Answer from the drawing. Dimensions are ordinates in mm from the lowest x, y and z of the part. Coordinates: 2 decimals unless noted, no trailing zeros. Write each loop counter-clockwise with the first axis right and the second up, starting at its lowest first coordinate (ties: lowest second). Pieces come first, ordered by that corner, then holes.
1) Determine the mould class of the marked faces 1, 2 and 3 for opening direction X: +X half, -X half, draft (parallel to the pull), parting line (faces both ways), or undercut.
2) The part is cut by section A-A (z = 1.75). Determine the outline of the cut face in (x, y).
3) Find the intervals of material crossed by line 1 (X direction, y = 0.25, z = 3.5) (1 decimal); line 2 (X direction, y = 1, z = 4); line 3 (Z direction, x = 3, y = 1.3) (1 decimal), in increasing order.
4) The part is cut by section D-D (z = 5.5). Determine the outline of the cut face in (x, y).
5) The part is cut by section B-B (x = 3.5). Determine the outline of the cut face in (y, z) (1 decimal).
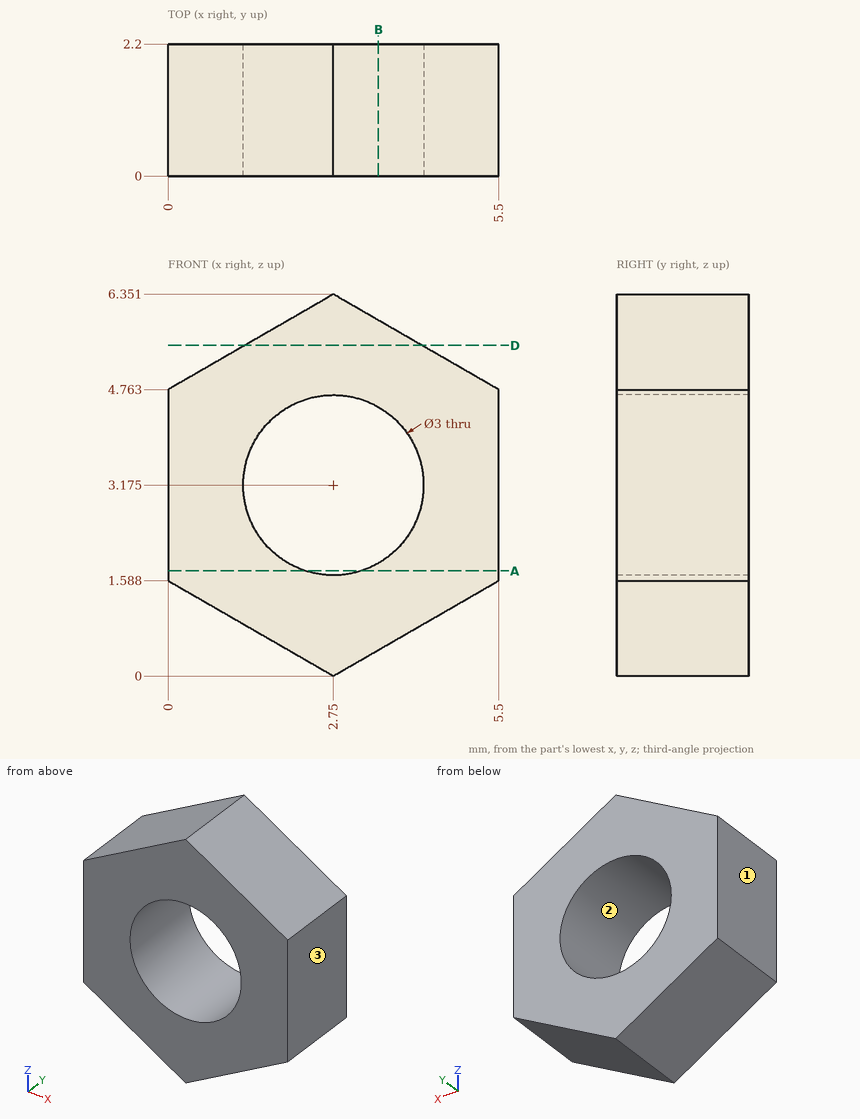
Reported:
1. face 1: -X half
1. face 2: undercut
1. face 3: +X half
2. outline: (0, 0) - (2.28, 0) - (2.28, 2.2) - (0, 2.2) - close; (3.22, 0) - (5.5, 0) - (5.5, 2.2) - (3.22, 2.2) - close
3. line 1: x = 0 to 1.3, 4.2 to 5.5
3. line 2: x = 0 to 1.5, 4 to 5.5
3. line 3: z = 0.1 to 1.7, 4.7 to 6.2
4. outline: (1.28, 0) - (4.22, 0) - (4.22, 2.2) - (1.28, 2.2) - close
5. outline: (0, 0.4) - (2.2, 0.4) - (2.2, 1.9) - (0, 1.9) - close; (0, 4.5) - (2.2, 4.5) - (2.2, 5.9) - (0, 5.9) - close
